Geometry: final body of the model. Coordinates: model frame, mm. Face numbers are marked on the shaded views. A direction names the side the tool comes from. Round coordinates to 2 decimals unless told otherwise and drop trailing zeros. Loops run counter-clockwise (first coordinate to the right, second up) from the corner with the lowest first, then second, coordinate; pieces in that order, holes last. Notation, with made-up numbers: (35, -39.5) - (72, -39.5) arc R10 ccw to (72, -24.5) - close; hole circle Ø1 at (21, 80.25). An arc over 180 degrees is marked (long way). Use CSV: the item, a comma, the result in double quotes.
from build123d import *

# Parameters (mm, degrees)
F0_W     = 100
F0_H     = 45
F1_DEPTH = 80
F3_DEPTH = 30
F5_DEPTH = 45.001
F6_DEPTH = 20
F4_W     = 20
F4_H     = 15
F7_DEPTH = 10


with BuildPart() as f1:
    # F0 (on Front) → F1 (new body)
    with BuildSketch(Plane.XZ):
        with Locations((-50, 22.5)):
            Rectangle(F0_W, F0_H)
    extrude(amount=F1_DEPTH)

    # F2 (on face) → F3 (cut)
    with BuildSketch(Plane.XY.offset(45)):
        with BuildLine():
            ThreePointArc((-32.5, -15), (-34.6966991411, -9.6966991411), (-40, -7.5))
            ThreePointArc((-40, -7.5), (-45.3033008589, -20.3033008589), (-32.5, -15))
        make_face()
    extrude(amount=-F3_DEPTH, mode=Mode.SUBTRACT)

    # F4 (on face) → F5 (cut, through all)
    with BuildSketch(Plane.XY.offset(45)):
        with BuildLine():
            Line((-57.3655851185, -50), (-36.7544467966, -50))
            ThreePointArc((-36.7544467966, -50), (-48.5464237678, -32.5391793906), (-65, -19.3782217351))
            Line((-65, -19.3782217351), (-65, -49.3667125702))
            Line((-65, -49.3667125702), (-65, -50))
            Line((-65, -50), (-57.3655851185, -50))
        make_face()
    extrude(amount=-F5_DEPTH, mode=Mode.SUBTRACT)

    # F4 (on face) → F6 (cut)
    with BuildSketch(Plane.XY.offset(45)):
        with BuildLine():
            Line((-80, -80), (-30, -80))
            ThreePointArc((-30, -80), (-31.7094855627, -64.6245117839), (-36.7544467966, -50))
            Line((-36.7544467966, -50), (-57.3655851185, -50))
            Line((-57.3655851185, -50), (-65, -50))
            Line((-65, -50), (-65, -49.3667125702))
            Line((-65, -49.3667125702), (-65, -19.3782217351))
            ThreePointArc((-65, -19.3782217351), (-81.8826668428, -12.3851921598), (-100, -10))
            Line((-100, -10), (-100, -65))
            Line((-100, -65), (-80, -65))
            Line((-80, -65), (-80, -80))
        make_face()
    extrude(amount=-F6_DEPTH, mode=Mode.SUBTRACT)

    # F4 (on face) → F7 (cut)
    with BuildSketch(Plane.XY.offset(45)):
        with Locations((-90, -72.5)):
            Rectangle(F4_W, F4_H)
    extrude(amount=-F7_DEPTH, mode=Mode.SUBTRACT)


solid = f1.part
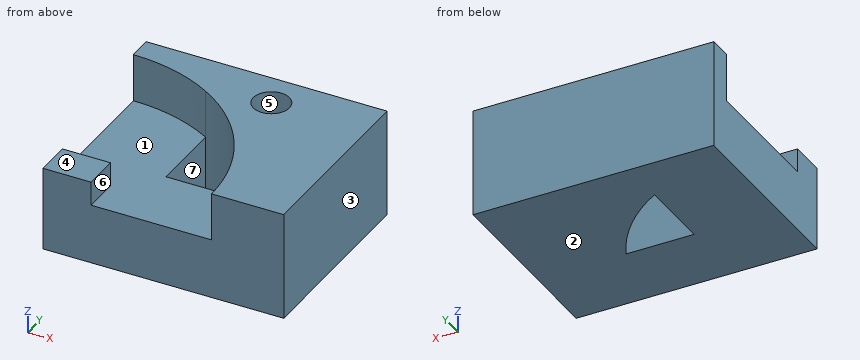
Item 1: Section A-A on z = 12. Return the cut outline in (x, y).
Final values:
outline,"(-100, -80) - (0, -80) - (0, 0) - (-100, 0) - close; hole (-65, -50) - (-36.75, -50) arc R70 ccw to (-65, -19.38) - close"
Item 2: Mould query, pull axis X, two halves, no side actions, for the marked faces 1, 2 and 3. Classes: released by +X, released by -X, zero draft, split by the parting line, or undercut.
Final values:
face 1,"undercut"
face 2,"zero draft"
face 3,"released by +X"
Item 3: Material intervals for line 1 (Y direction, x = -40, z = 24); line 2 (X direction, y = -24, z = 20); line 3 (Z direction, x = -53, y = -63), sorted ascending.
Final values:
line 1,"y = -80 to -50, -43.94 to -22.5, -7.5 to 0"
line 2,"x = -100 to -65, -58 to 0"
line 3,"z = 0 to 25"
Item 4: Section B-B on y = -34. Return the cut outline in (x, z), plus the area to 3 significant figures.
Final values:
outline,"(-100, 0) - (-65, 0) - (-65, 25) - (-100, 25) - close; (-47.24, 0) - (0, 0) - (0, 45) - (-47.24, 45) - close"
area,"3,000 mm²"
Item 5: Section D-D on z = 23.5. Return the cut outline in (x, y), plus the area to 3 significant figures.
Final values:
outline,"(-100, -80) - (0, -80) - (0, 0) - (-100, 0) - close; hole (-65, -50) - (-36.75, -50) arc R70 ccw to (-65, -19.38) - close; hole circle Ø15 at (-40, -15)"
area,"7,300 mm²"
Item 6: Pin query (flat end, axial travel): P1, Ø6, axis at x = -62, z = 32.5, coming from the -Y side; P2, Ø12, axis at x = -86.5, y = -70, coming from the +Z side; P3, Ø12, axis at x = -39, y = -15, coming from the +Z side. Return the tip coordinate at first contact, or that it passes through.
Final values:
P1,"stops at y = -23.26"
P2,"stops at z = 35"
P3,"stops at z = 15"
Item 7: Section C-C on x = -40. Return the cut outline in (y, z).
Final values:
outline,"(-80, 0) - (-50, 0) - (-50, 25) - (-80, 25) - close; (-43.94, 0) - (0, 0) - (0, 45) - (-7.5, 45) - (-7.5, 15) - (-22.5, 15) - (-22.5, 45) - (-43.94, 45) - close"
Item 8: Reachability of the marked faces 4, 5, 6 and 7 from +Z, -Z, +X, -X, +Y, -Y: full face, straight path, thin tool, end or side. Return the list, or none.
Final values:
face 4,"+Z, -X, -Y"
face 5,"+Z"
face 6,"+Z, -Y"
face 7,"+Z, -Z"
